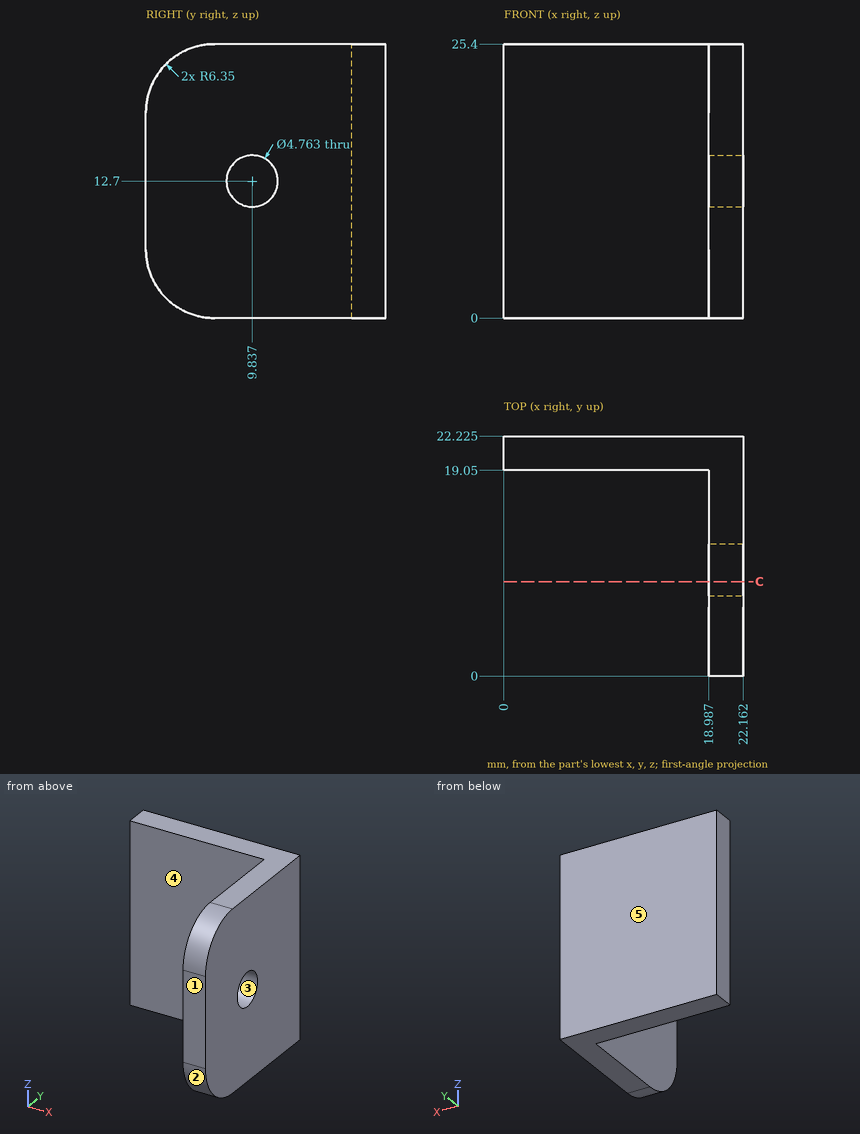
Part print with two shaded views. Sizes in mm from the minimum x, y, z corner. A direction names the side the tool comes from. Round coordinates to 2 decimals unless told otherwise and drop trailing zeros. Order: outer loops, then holes, each group sorted by start corner. A loop starts at its lowest first (then second) coordinate and runs counter-clockwise, first axis right, second up. Notation, with made-up numbers: M 31.5,13.5 L 36.5,13.5 A9 cw 36.5,25.5 Z; hole C -16,-0.75 d11. An arc over 180 degrees is marked long. Answer in a Markdown table with one row per item. Add a question column.
Q1. Mould opens along Z. For the marked faces 1, 2 and 3 say: +Z half, -Z half, draft (parallel to the pull), parting line (faces both ways), or undercut.
Q2. 3-axis set-ups, long thin cutter, end or side, ignore diameter. For the marked faces 4 and 5: which of +Z, -Z, +X, -X, +Y, -Y reach the whole face in a straight line?
Q3. Cut at C-C on y = 8.75. Give the cut face in (x, z).
Q4. Wall check: L1, parallel to X at y = 18, z = 2.75. Give the ranges that are in metal, low to high. Write a range as from..to.
Q5. Pin check, flat tips, straight feed: pin 1 (5.5 mm diameter, centred on y = 5.5, z = 15, fed in from -X); pin 2 (9.5 mm diameter, centred on x = 9.5, z = 9, fed in from -Y). Stop position of each tip, or through.
Established:
| question | item | result |
|---|---|---|
| 1 | face 1 | draft |
| 1 | face 2 | -Z half |
| 1 | face 3 | undercut |
| 2 | face 4 | +Z, -Z, -X, -Y |
| 2 | face 5 | +Z, -Z, +X, -X, +Y |
| 3 | outline | M 18.99,0 L 22.16,0 L 22.16,10.58 L 18.99,10.58 Z; M 18.99,14.82 L 22.16,14.82 L 22.16,25.4 L 18.99,25.4 Z |
| 4 | L1 | x = 18.99..22.16 |
| 5 | pin 1 | stops at x = 18.99 |
| 5 | pin 2 | stops at y = 19.05 |
